from build123d import *

# Parameters (mm, degrees)
F0_W     = 10
F0_H     = 3
F1_DEPTH = 23
F0_W_2   = 4
F2_DEPTH = 3
F4_DEPTH = 2
F6_DEPTH = 2
F7_R     = 1


with BuildPart() as f1:
    # F0 (on Top) → F1 (new body)
    with BuildSketch(Plane.XY):
        with Locations((21.8589810431, 48.6359097213)):
            Rectangle(F0_W, F0_H)
    extrude(amount=F1_DEPTH)



with BuildPart() as f1b:
    # F0 (on Top) → F1, piece 2 (new body)
    with BuildSketch(Plane.XY):
        with Locations((7.8589810431, 48.6359097213)):
            Rectangle(F0_W, F0_H)
    extrude(amount=F1_DEPTH)


with BuildPart() as f1c:
    # F0 (on Top) → F1, piece 3 (new body)
    with BuildSketch(Plane.XY):
        with Locations((7.8589810431, -21.3640902787)):
            Rectangle(F0_W, F0_H)
    extrude(amount=F1_DEPTH)


with BuildPart() as f1d:
    # F0 (on Top) → F1, piece 4 (new body)
    with BuildSketch(Plane.XY):
        with Locations((21.8589810431, -21.3640902787)):
            Rectangle(F0_W, F0_H)
    extrude(amount=F1_DEPTH)


with BuildPart() as f1_1:
    add(f1.part)

    add(f1b.part)  # F2 merges F1b

    add(f1c.part)  # F2 merges F1c

    add(f1d.part)  # F2 merges F1d
    # F0 (on Top) → F2 (join)
    with BuildSketch(Plane.XY):
        Polygon((12.8589810431, 47.1359097213), (2.8589810431, 47.1359097213), (2.8589810431, -19.8640902787), (12.8589810431, -19.8640902787), (16.8589810431, -19.8640902787), (26.8589810431, -19.8640902787), (26.8589810431, 47.1359097213), (16.8589810431, 47.1359097213), align=None)
        with Locations((14.8589810431, -21.3640902787)):
            Rectangle(F0_W_2, F0_H)
        with Locations((14.8589810431, 48.6359097213)):
            Rectangle(F0_W_2, F0_H)
    extrude(amount=F2_DEPTH)

    # F3 (on face) → F4 (join)
    with BuildSketch(Plane(origin=(2.8589810431, 0, 0), x_dir=(0, -1, 0), z_dir=(-1, 0, 0))):
        Polygon((19.8640902787, 23), (4.8640902787, 3), (19.8640902787, 3), align=None)
        Polygon((-32.1359097213, 3), (-47.1359097213, 23), (-47.1359097213, 3), align=None)
    extrude(amount=-F4_DEPTH)

    # F5 (on face) → F6 (join)
    with BuildSketch(Plane.YZ.offset(26.8589810431)):
        Polygon((47.1359097213, 23), (32.1359097213, 3), (47.1359097213, 3), align=None)
        Polygon((-4.8640902787, 3), (-19.8640902787, 23), (-19.8640902787, 3), align=None)
    extrude(amount=-F6_DEPTH)

    # F7
    f7_edges = [f1_1.edges().sort_by_distance(p)[0] for p in [
        (26.858981, 13.63591, 0),
        (14.858981, 50.13591, 0),
        (2.858981, 13.63591, 0),
        (14.858981, -22.86409, 0),
        (16.858981, -22.86409, 13),
        (21.858981, -22.86409, 23),
        (26.858981, -22.86409, 11.5),
        (2.858981, -22.86409, 11.5),
        (7.858981, -22.86409, 23),
        (12.858981, -22.86409, 13),
        (14.858981, -22.86409, 3),
        (12.858981, 50.13591, 13),
        (7.858981, 50.13591, 23),
        (2.858981, 50.13591, 11.5),
        (26.858981, 50.13591, 11.5),
        (21.858981, 50.13591, 23),
        (16.858981, 50.13591, 13),
        (14.858981, 50.13591, 3),
        (2.858981, -21.36409, 23),
        (2.858981, 48.63591, 23),
        (2.858981, 39.63591, 13),
        (2.858981, 13.63591, 3),
        (2.858981, -12.36409, 13),
        (26.858981, -21.36409, 23),
        (26.858981, -12.36409, 13),
        (26.858981, 13.63591, 3),
        (26.858981, 39.63591, 13),
        (26.858981, 48.63591, 23),
    ]]
    fillet(f7_edges, radius=F7_R)


solid = f1_1.part
The listing builds one solid part. Answer for the finished solid, in the listing's coordinates (mm). A direction names the side the tool comes from. Give positions to 0.01 mm unless a question says otherwise; leave off trailing zeros. Order: outer loops, then holes, each group sorted by start corner. A loop starts at its lowest first (then second) coordinate and runs counter-clockwise, first axis right, second up. Notation, with made-up numbers: (50.5, 47.5) - (67.5, 47.5) arc R27 ccw to (67.5, 68.5) - close; hole circle Ø4 at (11.25, 76). An arc over 180 degrees is marked (long way). One line per item, written item: value. Start each with the question number.
1) A tool of negligible diameter and unlimited length cuts with its end or side. For faces 1 (the face through (21, -19.864, 13)), 2 (the face through (12.859, 48, 13)), 3 (the face through (26.574, -12.562, 12.762)), from which of +Z, -Z, +X, -X, +Y, -Y can it reach the whole face along a straight path? Write none if from no direction.
2) A cutting plane is placed at D-D on x = 10.75. Give the vertices of the cut face in (y, z), then the cut area to 3 significant figures.
3) A cutting plane is placed at A-A on y = 20. Give the vertices of the cut face in (x, z), then the cut area to 3 significant figures.
4) A cutting plane is placed at B-B on x = 13.75. Give the vertices of the cut face in (y, z), then the cut area to 3 significant figures.
5) A cutting plane is placed at C-C on z = 7. State how many separate pieces and enclosed holes the cut face has, then the cut area to 3 significant figures.
6) Find the intervals of material crossed by L1, parallel to Y at x = 20, z = 14.5; L2, parallel to X at y = 37, z = 4.75; L3, parallel to Z at x = 11, y = 8, in increasing order.
7) The mould has two halves that part along Y. Classify faces 4 (the face through (15, 14, 0)), 5 (the face through (10, 50.136, 11)), 6 (the face through (9, 47.136, 13)), 7 (the face through (10, -22.864, 11)): released by +Y, released by -Y, zero draft, split by the parting line, or undercut.
8) Given pin 1 Ø10 at (x, y) = (21.5, 20.5) entering from +Z, flat-ended and moving along its own axis, determine where the tip first touches the part or whether it passes through.
Answer sheet:
1. face 1: +Z
1. face 2: +Z, +Y, -Y
1. face 3: +Z, +X
2. outline: (-22.86, 1) arc R1 ccw to (-21.86, 0) - (49.14, 0) arc R1 ccw to (50.14, 1) - (50.14, 22) arc R1 ccw to (49.14, 23) - (47.14, 23) - (47.14, 3) - (-19.86, 3) - (-19.86, 23) - (-21.86, 23) arc R1 ccw to (-22.86, 22) - close
2. area: 338 mm2
3. outline: (2.86, 1) arc R1 ccw to (3.86, 0) - (25.86, 0) arc R1 ccw to (26.86, 1) - (26.86, 2) arc R1 ccw to (25.86, 3) - (3.86, 3) arc R1 ccw to (2.86, 2) - close
3. area: 71.1 mm2
4. outline: (-22.86, 1) arc R1 ccw to (-21.86, 0) - (49.14, 0) arc R1 ccw to (50.14, 1) - (50.14, 2) arc R1 ccw to (49.14, 3) - (-21.86, 3) arc R1 ccw to (-22.86, 2) - close
4. area: 218 mm2
5. separate pieces: 4
5. enclosed holes: 0
5. area: 213 mm2
6. L1: y = -22.86 to -19.86, 47.14 to 50.14
6. L2: x = 2.86 to 4.86, 24.86 to 26.86
6. L3: z = 0 to 3
7. face 4: zero draft
7. face 5: released by +Y
7. face 6: undercut
7. face 7: released by -Y
8. pin 1: stops at z = 3
